Source: CAD feature listing. Evaluate the final solid. Frame: model axes, mm. Face numbers are marked on the shaded views. A direction names the side the tool comes from. Coordinates: 2 decimals unless noted, no trailing zeros. Write each loop counter-clockwise with the first axis right and the second up, starting at its lowest first coordinate (ties: lowest second). Pieces come first, ordered by that corner, then holes. Notation, with made-up numbers: M 42,-31.5 L 76,-31.5 A32 ccw 76,7.5 Z; hole C 67.25,-4.75 d3. An arc over 180 degrees is marked long. Answer as CSV lines item,"result". Start each with the question number.
1. Section A-A on x = 0. Count the separate pieces of the cut face and the enclosed holes in it, plus the area to 3 significant figures.
2. Section C-C on x = -3.5. Return the cut outline in (y, z).
3. Contact query for flat-ended pins moving along their axis: pin 1 Ø2 at (x, z) = (-3, 4) entering from -Y; pin 2 Ø5 at (x, z) = (7.5, 15.5) entering from +Y. Output: stop coordinate, or through.
4. Section B-B on y = 1.25. Return the cut outline in (x, z) (3 decimals), plus the area to 3 significant figures.
5. Mould query, pull axis Z, two halves, no side actions, for the marked faces 1, 2, 3 and 4. Classes: pulls with the +Z half, pulls with the -Z half, needs draft (parallel to the pull), parting line crosses it, or undercut.
6. Reachability of the marked faces 5 and 6 from +Z, -Z, +X, -X, +Y, -Y: full face, straight path, thin tool, end or side. Return the list, or none.
7. Line query: probe 1 along Z at (x, y) = (0, 1.7); probe 2 along Z at (x, y) = (4.5, 5.75); probe 3 along Z at (x, y) = (6, 1.5). Output: solid intervals per line, ascending. Write a range as [from, to].
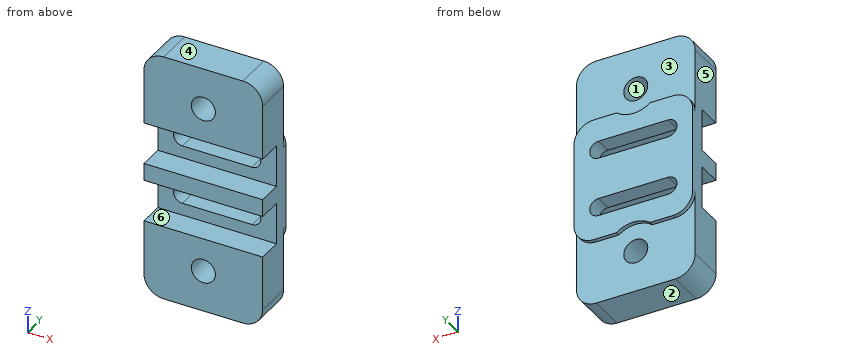
Autodesk Inventor part; units mm, degrees
ref_plane "XZ Plane" through (0, 0, 0) normal (0, 1, 0) x (-1, 0, 0)
sketch "Sketch1" plane through (0, 0, 0) normal (0, 1, 0) x (-1, 0, 0)
  line L0 (-9.525, 20.1041) -> (9.525, 20.1041)
  line L1 (9.525, 20.1041) -> (9.525, -20.1041)
  line L2 (9.525, -20.1041) -> (-9.525, -20.1041)
  line L3 (-9.525, -20.1041) -> (-9.525, 20.1041)
  line L4 (-9.525, 20.1041) -> (9.525, -20.1041) construction
  line L5 (9.525, 20.1041) -> (-9.525, -20.1041) construction
  line L6 (-5.3594, 9.9441) -> (5.3594, 9.9441) construction
  line L7 (5.3594, 9.9441) -> (5.3594, -9.9441) construction
  line L8 (5.3594, -9.9441) -> (-5.3594, -9.9441) construction
  line L9 (-5.3594, -9.9441) -> (-5.3594, 9.9441) construction
  line L10 (-5.3594, 9.9441) -> (5.3594, -9.9441) construction
  line L11 (5.3594, 9.9441) -> (-5.3594, -9.9441) construction
  circle A0 centre (0, 13.4747) radius 1.9304
  circle A1 centre (0, 13.4747) radius 4.445 construction
  circle A2 centre (0, -13.4747) radius 1.9304
  circle A3 centre (0, -13.4747) radius 4.445 construction
  line L12 (9.525, 0) -> (-9.525, 0) construction
  point P0 (0, 0)
  dimension "d0" = 19.05
  dimension "d1" = 40.2082
  dimension "d2" = 10.7188
  dimension "d3" = 19.8882
  dimension "d5" = 3.8608
  dimension "d7" = 8.89
  dimension "d8" = 3.8608
  dimension "d10" = 8.89
  dimension "d33" = 26.9494
extrude "TNutMount" add sketch "Sketch1" along normal blind 5.9436
sketch "Sketch2" plane through (0, 5.9436, 0) normal (0, 1, 0) x (1, 0, 0)
  line L0 (-9.525, -9.9441) -> (9.525, -9.9441)
  line L1 (9.525, -9.9441) -> (9.525, 9.9441)
  line L2 (9.525, 9.9441) -> (-9.525, 9.9441)
  line L3 (-9.525, 9.9441) -> (-9.525, -9.9441)
  line L4 (-9.525, -9.9441) -> (9.525, 9.9441) construction
  line L5 (9.525, -9.9441) -> (-9.525, 9.9441) construction
  point P0 (0, 0)
  dimension "d13" = 19.05
  dimension "d14" = 19.8882
extrude "SwitchMount" add sketch "Sketch2" along normal blind 0.6858
sketch "Sketch3" plane through (0, 6.6294, 0) normal (0, 1, 0) x (1, 0, 0)
  line L0 (5.588, -4.7625) -> (-5.588, -4.7625) construction
  line L1 (-5.588, -4.7625) -> (-5.588, 4.7625) construction
  line L2 (-5.588, 4.7625) -> (5.588, 4.7625) construction
  line L3 (5.588, 4.7625) -> (5.588, -4.7625) construction
  line L4 (5.588, -4.7625) -> (-5.588, 4.7625) construction
  line L5 (-5.588, -4.7625) -> (5.588, 4.7625) construction
  line L6 (-5.588, 4.7625) -> (5.588, 4.7625) construction
  line L7 (-5.588, 3.3528) -> (5.588, 3.3528)
  line L8 (5.588, 6.1722) -> (-5.588, 6.1722)
  arc A0 (-5.588, 6.1722) -> (-5.588, 3.3528) centre (-5.588, 4.7625) ccw
  arc A1 (5.588, 3.3528) -> (5.588, 6.1722) centre (5.588, 4.7625) ccw
  line L9 (-5.588, -4.7625) -> (5.588, -4.7625) construction
  line L10 (-5.588, -6.1722) -> (5.588, -6.1722)
  line L11 (5.588, -3.3528) -> (-5.588, -3.3528)
  arc A2 (-5.588, -3.3528) -> (-5.588, -6.1722) centre (-5.588, -4.7625) ccw
  arc A3 (5.588, -6.1722) -> (5.588, -3.3528) centre (5.588, -4.7625) ccw
  point P0 (0, 0)
  point P1 (0, 4.7625)
  point P2 (0, -4.7625)
  dimension "d19" = 11.176
  dimension "d20" = 9.525
  dimension "d21" = 2.8194
  dimension "d22" = 2.8194
extrude "ScrewSlot" cut sketch "Sketch3" against normal through all
sketch "Sketch4" plane through (0, 0, 0) normal (0, -1, 0) x (1, 0, 0)
  arc A0 (5.588, -6.1722) -> (5.588, -3.3528) centre (5.588, -4.7625) ccw
  arc A1 (-5.588, -3.3528) -> (-5.588, -6.1722) centre (-5.588, -4.7625) ccw
  line L0 (5.588, -4.7625) -> (-5.588, -4.7625) construction
  arc A2 (5.588, 3.3528) -> (5.588, 6.1722) centre (5.588, 4.7625) ccw construction
  arc A3 (-5.588, 6.1722) -> (-5.588, 3.3528) centre (-5.588, 4.7625) ccw construction
  line L1 (5.588, 4.7625) -> (-5.588, 4.7625) construction
  line L2 (-9.525, -1.397) -> (9.525, -1.397)
  line L3 (9.525, -1.397) -> (9.525, -8.128)
  line L4 (9.525, -8.128) -> (-9.525, -8.128)
  line L5 (-9.525, -8.128) -> (-9.525, -1.397)
  line L6 (-9.525, -1.397) -> (9.525, -8.128) construction
  line L7 (9.525, -1.397) -> (-9.525, -8.128) construction
  line L8 (-9.525, 8.128) -> (9.525, 8.128)
  line L9 (9.525, 8.128) -> (9.525, 1.397)
  line L10 (9.525, 1.397) -> (-9.525, 1.397)
  line L11 (-9.525, 1.397) -> (-9.525, 8.128)
  line L12 (-9.525, 8.128) -> (9.525, 1.397) construction
  line L13 (9.525, 8.128) -> (-9.525, 1.397) construction
  point P0 (0, 0)
  point P1 (0, -4.7625)
  point P2 (0, 4.7625)
  dimension "d25" = 19.05
  dimension "d26" = 6.731
  dimension "d27" = 19.05
  dimension "d28" = 6.731
extrude "Extrusion4" cut sketch "Sketch4" against normal blind 3.937
fillet "Fillet1" radius 3.175 8 edges at (9.525, 2.9718, 20.1041) (9.525, 2.9718, -20.1041) (-9.525, 2.9718, 20.1041) (-9.525, 2.9718, -20.1041) (9.525, 6.2865, -9.9441) (9.525, 6.2865, 9.9441) (-9.525, 6.2865, -9.9441) (-9.525, 6.2865, 9.9441)
sketch "Sketch5" plane through (0, 5.9436, 0) normal (0, 1, 0) x (1, 0, 0)
  circle A0 centre (0, 13.4747) radius 1.9304
  circle A1 centre (0, 13.4747) radius 4.445
  circle A2 centre (0, -13.4747) radius 1.9304
  circle A3 centre (0, -13.4747) radius 4.445
  point P0 (0, 0)
  dimension "d36" = 8.89
  dimension "d37" = 8.89
extrude "Extrusion5" cut sketch "Sketch5" along normal up to surface (0.6858 mm away)
properties part number "limit switch mount to xrail"
Values:
1,separate pieces,"5"
1,enclosed holes,"0"
1,area,"137 mm²"
2,outline,"M 0,-20.1 L 5.94,-20.1 L 5.94,-9.94 L 6.63,-9.94 L 6.63,-6.17 L 3.94,-6.17 L 3.94,-8.13 L 0,-8.13 Z; M 0,-1.4 L 3.94,-1.4 L 3.94,-3.35 L 6.63,-3.35 L 6.63,3.35 L 3.94,3.35 L 3.94,1.4 L 0,1.4 Z; M 0,8.13 L 3.94,8.13 L 3.94,6.17 L 6.63,6.17 L 6.63,9.94 L 5.94,9.94 L 5.94,20.1 L 0,20.1 Z"
3,pin 1,"y = 3.94"
3,pin 2,"y = 5.94"
4,outline,"M -9.525,-16.929 A3.175 ccw -6.35,-20.104 L 6.35,-20.104 A3.175 ccw 9.525,-16.929 L 9.525,-8.128 L -9.525,-8.128 Z; M -9.525,-1.397 L 9.525,-1.397 L 9.525,1.397 L -9.525,1.397 Z; M -9.525,8.128 L 9.525,8.128 L 9.525,16.929 A3.175 ccw 6.35,20.104 L -6.35,20.104 A3.175 ccw -9.525,16.929 Z; hole C 0,-13.475 d3.861; hole C 0,13.475 d3.861"
4,area,"477 mm²"
5,face 1,"undercut"
5,face 2,"pulls with the -Z half"
5,face 3,"needs draft"
5,face 4,"pulls with the +Z half"
6,face 5,"+Z, -Z, -X, +Y, -Y"
6,face 6,"+X, -X, -Y"
7,probe 1,"[-20.1, -15.41], [-11.54, -8.13], [-1.4, 1.4], [8.13, 11.54], [15.41, 20.1]"
7,probe 2,"[-20.1, -6.17], [-3.35, 3.35], [6.17, 20.1]"
7,probe 3,"[-20.1, -8.13], [-1.4, 1.4], [8.13, 20.1]"
